Could you check a few things on this model? Use its own coordinates, in mm. A direction names the side the tool comes from. Give positions to 0.01 mm unless a question says otherwise; leave off trailing zeros. Write each loop counter-clockwise with the first axis right and the second up, starting at its lowest first coordinate (ties: lowest second). Pieces come first, ordered by that corner, then holes. Notation, with made-up numbers: (60.25, -23.5) - (107.25, -23.5) arc R23 cw to (107.25, -1.5) - close; hole circle Ø11 at (17.25, -17). An arc over 180 degrees is marked (long way). Answer in a Markdown table with one row per item.
from build123d import *

# Parameters (mm, degrees)
SKETCH1_W                     = 33
SKETCH1_H                     = 10
BOSS_EXTRUDE1_DEPTH           = 3
CSK_FOR_M3_SFHCS1_D           = 3.4
CSK_FOR_M3_SFHCS1_DEPTH       = 10
CSK_FOR_M3_SFHCS1_CSINK_D     = 6.72
CSK_FOR_M3_SFHCS1_CSINK_ANGLE = 90
CSK_FOR_M3_SFHCS1_TIP         = 1.021463052
FILLET1_R                     = 4


with BuildPart() as part:
    # Sketch1 → Boss-Extrude1 (new body)
    with BuildSketch(Plane(origin=(0, 0, 0), x_dir=(1, 0, 0), z_dir=(0, 1, 0))):
        with Locations((0, -5)):
            Rectangle(SKETCH1_W, SKETCH1_H)
        with BuildLine():
            Line((-4, 0), (-2.5, 0))
            Line((-2.5, 0), (-2.5, 10))
            Line((-2.5, 10), (-4, 10))
            ThreePointArc((-4, 10), (-4.267949192, 9), (-5, 8.267949192))
            ThreePointArc((-5, 8.267949192), (-6, 6.535898385), (-5, 4.803847577))
            ThreePointArc((-5, 4.803847577), (-4.267949192, 4.07179677), (-4, 3.07179677))
            Line((-4, 3.07179677), (-4, 0))
        make_face()
        with BuildLine():
            Line((2.5, 10), (2.5, 0))
            Line((2.5, 0), (4, 0))
            Line((4, 0), (4, 3.07179677))
            ThreePointArc((4, 3.07179677), (4.267949192, 4.07179677), (5, 4.803847577))
            ThreePointArc((5, 4.803847577), (6, 6.535898385), (5, 8.267949192))
            ThreePointArc((5, 8.267949192), (4.267949192, 9), (4, 10))
            Line((4, 10), (2.5, 10))
        make_face()
    extrude(amount=BOSS_EXTRUDE1_DEPTH)

    # CSK for M3 SFHCS1
    with Locations(Plane(origin=(0, 3, 0), x_dir=(1, 0, 0), z_dir=(0, 1, 0))):
        with Locations((-12.5, -6), (12.5, -6)):
            CounterSinkHole(CSK_FOR_M3_SFHCS1_D / 2, CSK_FOR_M3_SFHCS1_CSINK_D / 2, depth=CSK_FOR_M3_SFHCS1_DEPTH, counter_sink_angle=CSK_FOR_M3_SFHCS1_CSINK_ANGLE)
            with Locations((0, 0, -(CSK_FOR_M3_SFHCS1_DEPTH + CSK_FOR_M3_SFHCS1_TIP / 2))):  # 118° drill point
                Cone(0, CSK_FOR_M3_SFHCS1_D / 2, CSK_FOR_M3_SFHCS1_TIP, mode=Mode.SUBTRACT)

    # Fillet1
    fillet1_edges = [part.edges().sort_by_distance(p)[0] for p in [
        (16.5, 1.5, 10),
        (-16.5, 1.5, 10),
    ]]
    fillet(fillet1_edges, radius=FILLET1_R)


solid = part.part
1) We'd pull the mould along X, two halves only. Please class faces 1 (the face through (15.359, 1.521, 8.797)), 2 (the face through (-14.07, 0.66, 6.65)), 3 (the face through (0, 3, 2)): +X half, -X half, draft (parallel to the pull), parting line (faces both ways), or undercut.
Check values:
| item | result |
|---|---|
| face 1 | +X half |
| face 2 | undercut |
| face 3 | draft |
2) If I drill on line 1 (Z direction, x = 12.5, y = 0.55); line 2 (X direction, y = 0.5, z = -1); line 3 (X direction, y = 0.5, z = 5), over which ranges is the centre line in solid material (lowest first)?
Check values:
| item | result |
|---|---|
| line 1 | z = 0 to 4.3, 7.7 to 10 |
| line 2 | x = -4 to -2.5, 2.5 to 4 |
| line 3 | x = -16.5 to -13.87, -11.13 to 11.13, 13.87 to 16.5 |
3) Imagine slicing it at A-A (z = -7.25). List the corners of the cut face in (x, y) for me, then the cut area to 3 significant figures.
Check values:
| item | result |
|---|---|
| outline | (-5.87, 0) - (-2.5, 0) - (-2.5, 3) - (-5.87, 3) - close; (2.5, 0) - (5.87, 0) - (5.87, 3) - (2.5, 3) - close |
| area | 20.2 mm2 |
4) On a 3-axis mill with a long thin cutter (end or side, diameter ignored), from which of +Z, -Z, +X, -X, +Y, -Y can I reach the whole of each face in a straight line? I mean faces 4 (the face through (4, 1, -2)), 5 (the face through (3, 1, -10)), 6 (the face through (-4, 1, -2)), 7 (the face through (-16.5, 1, 3)), 8 (the face through (2.5, 1, -5)). Say none if no direction works.
Check values:
| item | result |
|---|---|
| face 4 | +X, +Y, -Y |
| face 5 | -Z, +X, -X, +Y, -Y |
| face 6 | -X, +Y, -Y |
| face 7 | +Z, -Z, -X, +Y, -Y |
| face 8 | -Z, +Y, -Y |
5) Imagine slicing it at B-B (y = 2.4). List the corners of the cut face in (x, z) for me.
Check values:
| item | result |
|---|---|
| outline | (-16.5, 0) - (-4, 0) - (-4, -3.07) arc R2 cw to (-5, -4.8) arc R2 ccw to (-5, -8.27) arc R2 cw to (-4, -10) - (-2.5, -10) - (-2.5, 0) - (2.5, 0) - (2.5, -10) - (4, -10) arc R2 cw to (5, -8.27) arc R2 ccw to (5, -4.8) arc R2 cw to (4, -3.07) - (4, 0) - (16.5, 0) - (16.5, 6) arc R4 ccw to (12.5, 10) - (-12.5, 10) arc R4 ccw to (-16.5, 6) - close; hole circle Ø5.52 at (-12.5, 6); hole circle Ø5.52 at (12.5, 6) |
6) Will these pins go through, and if not, where does the flat tip stop? P1, Ø4.5, axis at x = 12.5, z = 6, coming from the +Y side; P2, Ø0.9, axis at y = 2, z = -6, coming from the +X side; P3, Ø1, axis at y = 0.5, z = -3, coming from the +X side; P4, Ø1.5, axis at x = 12.5, z = -2.5, coming from the +Y side.
Check values:
| item | result |
|---|---|
| P1 | stops at y = 1.89 |
| P2 | stops at x = 6 |
| P3 | stops at x = 4.05 |
| P4 | passes through |
